Autodesk Inventor part; units mm, degrees
ref_plane "MSC_PF1" through (0, 0, 0) normal (1, 0, 0) x (0, 1, 0)
ref_plane "MSC_PT1" through (0, 0, 0) normal (0, 0, -1) x (-1, 0, 0)
ref_plane "YZ Plane" through (0, 0, 0) normal (1, 0, 0) x (0, 1, 0)
sketch "Esquisse1" plane through (0, 0, 0) normal (0, 1, 0) x (-1, 0, 0)
  point P0 (0, 0)
sketch "Esquisse2" plane through (0, 0, 0) normal (0, 0, 1) x (1, 0, 0)
  point P0 (0, 0)
sketch "Esquisse3" plane through (0, 0, 0) normal (0, 0, 1) x (1, 0, 0)
  point P0 (0, 0)
sketch "Esquisse4" plane through (0, 0, 0) normal (0, 1, 0) x (-1, 0, 0)
  line L0 (-2.35, 0) -> (0, 0)
  line L1 (-2.35, -0.4) -> (-2.35, 0)
  line L2 (-1.25, -1.5) -> (-2.35, -0.4)
  line L3 (-1.25, -1.725) -> (-1.25, -1.5)
  line L4 (-1.025, -1.95) -> (-1.25, -1.725)
  line L5 (-1.25, -2.175) -> (-1.025, -1.95)
  line L6 (-1.25, -8) -> (-1.25, -2.175)
  line L7 (0, 0) -> (0, -8)
  line L8 (0, 3.3392) -> (0, -10.7) construction
  line L9 (0, 3.3392) -> (0, -10.7)
  line L10 (0, -13.5078) -> (0, 6.1471)
  line L11 (-1.25, -8) -> (0, -8)
  line L12 (0.47, 0) -> (-2.82, 0)
  dimension "d3" = 2.35
  dimension "d5" = 0.225
  dimension "d7" = 0.225
  dimension "d9" = 0.225
  dimension "d11" = 1.5
  dimension "d13" = 135
  dimension "d17" = 1.025
  dimension "d19" = 0
  dimension "d51" = 1.25
  dimension "d52" = 8
revolve "Révolution1" add sketch "Esquisse4" angle 360 about axis through (0, 0, 3.3392) along (0, 0, -1)
sketch "Esquisse5" plane through (0, 0, 0) normal (0, 1, 0) x (-1, 0, 0)
  line L0 (-1.45, 0) -> (0, 0)
  line L1 (-0.2417, -1.3636) -> (-1.45, 0)
  line L2 (0, -1.3636) -> (-0.2417, -1.3636)
  line L3 (0, 0) -> (0, -1.3636)
  line L4 (-1.25, -1.5) -> (1.25, -1.5) construction
  line L5 (-2.35, 0) -> (2.35, 0)
  line L6 (0, -1.8) -> (0, 0.3)
  dimension "d22" = 1.45
  dimension "d24" = 0.2417
  dimension "d26" = 1.3636
extrude "Extrusion1" cut sketch "Esquisse5" along normal mid plane 0.4833
pattern_circular "RéseauPolaire1" count 4 over 360 about axis through (0, 0, 0) along (0, 0, 1) of "Extrusion1"
sketch "Esquisse7" plane through (0, 0, 0) normal (0, 1, 0) x (-1, 0, 0)
  line L0 (0, -0.75) -> (-1.8125, 0)
  line L1 (0, 0) -> (0, -0.75)
  line L2 (-1.8125, 0) -> (0, 0)
  line L3 (-1.25, -1.5) -> (1.25, -1.5) construction
  line L4 (0, -1.8) -> (0, 0.3)
  line L5 (-2.35, 0) -> (2.35, 0)
  dimension "d33" = 1.8125
  dimension "d35" = 0.75
extrude "Extrusion2" cut sketch "Esquisse7" along normal mid plane 0.4833
pattern_circular "RéseauPolaire2" count 4 over 360 about axis through (0, 0, 0) along (0, 0, 1) of "Extrusion2"
fillet "Congé1" radius 0.45 1 edges at (-1.25, 0, -1.5)
thread "Filetage1"
ref_plane "MSC_PF1" through (0, 0, 0) normal (1, 0, 0) x (0, 1, 0)
ref_plane "MSC_PT1" through (0, 0, 0) normal (0, 0, -1) x (-1, 0, 0)
equation "\"d3\" = 0.5 * Dh"
equation "\"d5\" = msp_x"
equation "\"d7\" = ParA"
equation "\"d9\" = msp_x"
equation "\"d11\" = ParK"
equation "\"d17\" = 0.5 * msp_mdtds"
equation "\"d51\" = 0.5 * NND"
equation "\"d52\" = NLG"
equation "\"d22\" = 0.5 * M"
equation "\"d24\" = 0.0833333 * M"
equation "\"d26\" = 0.909091 * ParK"
equation "\"d27\" = 0.166667 * M"
equation "\"d33\" = 0.625 * M"
equation "\"d35\" = 0.5 * ParK"
equation "\"d36\" = 0.166667 * M"
equation "\"d41\" = 2 * msp_x"
equation "\"PTC\" = 0.45"
equation "\"NLG\" = 8"
equation "\"ParK\" = 1.5"
equation "\"NND\" = 2.5"
equation "\"M\" = 2.9"
equation "\"msp_mdtds\" = NND - PTC"
equation "\"Dh\" = 4.7"
equation "\"msp_x\" = 0.5 * PTC"
equation "\"ParA\" = 0.5 * PTC"
equation "\"r\" = 0.6"
equation "\"THREADDIA\" = NND"
equation "\"TEMPLATE\" = 1.2345"
properties part number "NF EN ISO 7046-2 H - M2.5x8 - 8.8 - H1" material "Acier inoxydable 440C"
Input: part model. Units: mm. Frame: model coordinates. A direction names the side the tool comes from. Give positions to 0.01 mm unless a question says otherwise; leave off trailing zeros. Order: outer loops, then holes, each group sorted by start corner. A loop starts at its lowest first (then second) coordinate and runs counter-clockwise, first axis right, second up.
1. Set-up query: faces 1 (the face through (-0.242, 0.7, -0.4)), 2 (the face through (0, 0, -8)). Return all of +Z, -Z, +X, -X, +Y, -Y with unobstructed straight access to the full face (end or side cutting, diameter ignored); none if empty.
Computed:
face 1: +Z
face 2: -Z, +X, -X, +Y, -Y
2. Cut plane A-A (z = -3.25). Return loops of the section in (x, y).
Computed:
outline: circle Ø2.5 at (0, 0)
3. Draft query along X for faces 3 (the face through (0.7, -0.242, -0.4)), 4 (the face through (-0.27, -1.22, -5.05)), 5 (the face through (0.5, 0.5, 0)). Return one class per face: released by +X, released by -X, zero draft, split by the parting line, or undercut.
Computed:
face 3: undercut
face 4: split by the parting line
face 5: zero draft
4. Pin query (flat end, axial travel): pin 1 Ø1.1 at (y, z) = (-1, -0.5) entering from -X; pin 2 Ø0.7 at (y, z) = (1.5, -0.5) entering from -X; pin 3 Ø1.1 at (x, z) = (-1, -0.5) entering from -Y. Return the tip coordinate at first contact, or that it passes through.
Computed:
pin 1: stops at x = -2.3
pin 2: stops at x = -2.04
pin 3: stops at y = -2.3
5. Line query: probe 1 along Z at (x, y) = (-0.9, -1.05); probe 2 along Z at (x, y) = (-1.65, 0.7); probe 3 along Y at (x, z) = (0.2, -6.75). Output: solid intervals per line, ascending.
Computed:
probe 1: z = -1.37 to 0
probe 2: z = -0.96 to 0
probe 3: y = -1.23 to 1.23
